```python
from build123d import *

# Parameters (mm, degrees)
F1_DEPTH = 99.06
F2_SIZE  = 1.27
F3_SIZE  = 1.27


with BuildPart() as f1:
    # F0 (on Top) → F1 (new body)
    with BuildSketch(Plane.XY):
        Polygon((1.5875, -2.749631), (3.175, 0), (1.5875, 2.749631), (-1.5875, 2.749631), (-3.175, 0), (-1.5875, -2.749631), align=None)
    extrude(amount=F1_DEPTH)

    # F2
    f2_edges = [f1.edges().sort_by_distance(p)[0] for p in [
        (0, -2.749631, 99.06),
        (2.38125, -1.374815, 99.06),
        (2.38125, 1.374815, 99.06),
        (0, 2.749631, 99.06),
        (-2.38125, 1.374815, 99.06),
        (-2.38125, -1.374815, 99.06),
    ]]
    chamfer(f2_edges, length=F2_SIZE)

    # F3
    f3_edges = [f1.edges().sort_by_distance(p)[0] for p in [
        (0, -2.749631, 0),
        (2.38125, -1.374815, 0),
        (2.38125, 1.374815, 0),
        (0, 2.749631, 0),
        (-2.38125, 1.374815, 0),
        (-2.38125, -1.374815, 0),
    ]]
    chamfer(f3_edges, length=F3_SIZE)


solid = f1.part
```
Here's how the part is built. I have some questions about the finished solid (model axes, mm). Give positions to 0.01 mm unless a question says otherwise; leave off trailing zeros. Order: outer loops, then holes, each group sorted by start corner. A loop starts at its lowest first (then second) coordinate and runs counter-clockwise, first axis right, second up. Notation, with made-up numbers: (-0.5, -23) - (54.5, -23) arc R18 ccw to (54.5, -1) - close; hole circle Ø10 at (-14, 55). An arc over 180 degrees is marked (long way). Answer as a JSON object with one key per item and string values. Group by question number.
Item 1: For P1, Ø1, axis at y = 1.5, z = 35, coming from the -X side, with a flat end and sliding along its axis, tell me the tip position at first contact or that it passes through.
Item 2: If we section it at A-A on z = 82.5: Please give me the cut outline in (x, y) (1 decimal).
Item 3: Please list where these lines run through material, in increasing order: probe 1 along X at (y, z) = (2.55, 41); probe 2 along X at (y, z) = (-0.75, 46); probe 3 along Y at (x, z) = (3, 30.5).
Result set:
{
 "1": {"P1": "x = -2.6"},
 "2": {"outline": "(-3.2, 0) - (-1.6, -2.7) - (1.6, -2.7) - (3.2, 0) - (1.6, 2.7) - (-1.6, 2.7) - close"},
 "3": {"probe 1": "-1.7 to 1.7", "probe 2": "-2.74 to 2.74", "probe 3": "-0.3 to 0.3"}
}
